The model under review builds one solid part; all positions refer to its coordinate system, in mm. A direction names the side the tool comes from. Round coordinates to 2 decimals unless told otherwise and drop trailing zeros. Order: outer loops, then holes, each group sorted by start corner. A loop starts at its lowest first (then second) coordinate and runs counter-clockwise, first axis right, second up. Notation, with made-up numbers: (24.25, 69.5) -> (76.25, 69.5) arc R30 ccw to (76.25, 96.5) -> close; hole circle Ø1 at (62, -34). An arc over 180 degrees is marked (long way). Use a Markdown table: item, result. Add a question column.
```python
from build123d import *

# Parameters (mm, degrees)
F0_R     = 3.125
F0_R_2   = 3.2
F1_DEPTH = 6.2
F2_R     = 3.125
F3_DEPTH = 6


with BuildPart() as f1:
    # F0 (on Top) → F1 (new body)
    with BuildSketch(Plane.XY):
        with BuildLine():
            Line((11, -29.5), (11, 0))
            ThreePointArc((11, 0), (0.767321, 10.973205), (-10.892949, 1.530904))
            Line((-10.892949, 1.530904), (-24.61524, -96.108269))
            ThreePointArc((-24.61524, -96.108269), (-22.259655, -104.06059), (-14.712559, -107.5))
            Line((-14.712559, -107.5), (20.38476, -107.5))
            ThreePointArc((20.38476, -107.5), (27.455828, -104.571068), (30.38476, -97.5))
            Line((30.38476, -97.5), (30.38476, -39.5))
            ThreePointArc((30.38476, -39.5), (28.920294, -35.964466), (25.38476, -34.5))
            Line((25.38476, -34.5), (16, -34.5))
            ThreePointArc((16, -34.5), (12.464466, -33.035534), (11, -29.5))
        make_face()
        with BuildLine():
            Line((-18.875, -98.65), (-18.875, -94))
            ThreePointArc((-18.875, -94), (-14, -89.125), (-9.125, -94))
            Line((-9.125, -94), (-9.125, -98.65))
            ThreePointArc((-9.125, -98.65), (-14, -103.525), (-18.875, -98.65))
        make_face(mode=Mode.SUBTRACT)
        with Locations((22, -55)):
            Circle(F0_R, mode=Mode.SUBTRACT)
        Circle(F0_R_2, mode=Mode.SUBTRACT)
    extrude(amount=F1_DEPTH)

    # F2 (on face) → F3 (join)
    with BuildSketch(Plane.XY.offset(6.2)):
        with BuildLine():
            ThreePointArc((29.5, -52.875), (22, -45.375), (14.5, -52.875))
            Line((14.5, -52.875), (14.5, -57.125))
            ThreePointArc((14.5, -57.125), (22, -64.625), (29.5, -57.125))
            Line((29.5, -57.125), (29.5, -52.875))
        make_face()
        with Locations((22, -55)):
            Circle(F2_R, mode=Mode.SUBTRACT)
    extrude(amount=F3_DEPTH)


solid = f1.part
```
Q1. Draft analysis for pull direction Y (two halves, no side actions). For faces 1 (the face through (-9.125, -96, 3)), 2 (the face through (-18.875, -96, 3)), 3 (the face through (28.959, -36.004, 3.057)), 4 (the face through (30.385, -69, 3)), state which applies: released by +Y, released by -Y, zero draft, split by the parting line, or undercut.
Q2. For faces 5 (the face through (21.835, -64.623, 9.158)), 6 (the face through (22.165, -45.377, 9.158)), 7 (the face through (21, -34.5, 3)), list the 3-axis set-ups (+Z, -Z, +X, -X, +Y, -Y) from which the entire face can be reached by the end or side of a thin tool; tool diameter is ignored.
Q3. Add section A-A, the plane x = 0. Give the boundary of the cut face in (y, z), then the cut area to 3 significant figures.
Q4. Add section B-B, the plane y = -100. Give the boundary of the cut face in (x, z), then the cut area to 3 significant figures.
Q5. Add section C-C, the plane z = 10.25. Give the boundary of the cut face in (x, y) (3 decimals), then the cut area to 3 significant figures.
Q6. Add section D-D, the plane y = -48.5. Give the boundary of the cut face in (x, z), then the cut area to 3 significant figures.
Q7. To check wall thickness, follow line 1 along Y through (x, z) = (22, 9.5) (3 decimals); line 2 along Y through (x, z) = (0, 4.75); line 3 along Z through (x, y) = (10.5, -48). State the ranges of each line that lie inside material, in increasing order.
Q8. For pin 1 (8 mm diameter, centred on x = -6.5, y = -2, fed in from +Z); pin 2 (5 mm diameter, centred on y = -45, z = 2, fed in from -X); pin 3 (4.5 mm diameter, centred on y = -55.5, z = 10, fed in from +X), all flat-tipped, find the tip position at first contact; note any pin that passes through.
Return value:
| question | item | result |
|---|---|---|
| 1 | face 1 | undercut |
| 1 | face 2 | undercut |
| 1 | face 3 | released by +Y |
| 1 | face 4 | zero draft |
| 2 | face 5 | +Z, -Y |
| 2 | face 6 | +Z, +Y |
| 2 | face 7 | +Z, -Z, +X, +Y |
| 3 | outline | (-107.5, 0) -> (-3.2, 0) -> (-3.2, 6.2) -> (-107.5, 6.2) -> close; (3.2, 0) -> (11, 0) -> (11, 6.2) -> (3.2, 6.2) -> close |
| 3 | area | 695 mm² |
| 4 | outline | (-24.4, 0) -> (-18.68, 0) -> (-18.68, 6.2) -> (-24.4, 6.2) -> close; (-9.32, 0) -> (30.07, 0) -> (30.07, 6.2) -> (-9.32, 6.2) -> close |
| 4 | area | 280 mm² |
| 5 | outline | (14.5, -57.125) arc R7.5 ccw to (29.5, -57.125) -> (29.5, -52.875) arc R7.5 ccw to (14.5, -52.875) -> close; hole circle Ø6.25 at (22, -55) |
| 5 | area | 210 mm² |
| 6 | outline | (-17.92, 0) -> (30.38, 0) -> (30.38, 6.2) -> (28.09, 6.2) -> (28.09, 12.2) -> (15.91, 12.2) -> (15.91, 6.2) -> (-17.92, 6.2) -> close |
| 6 | area | 373 mm² |
| 7 | line 1 | -64.625 to -58.125, -51.875 to -45.375 |
| 7 | line 2 | -107.5 to -3.2, 3.2 to 11 |
| 7 | line 3 | 0 to 6.2 |
| 8 | pin 1 | z = 6.2 |
| 8 | pin 2 | x = -17.78 |
| 8 | pin 3 | x = 29.5 |
